```python
from build123d import *


with BuildPart() as part:
    # Sketch1 → Revolve1 (revolve)
    with BuildSketch(Plane.XY):
        with BuildLine():
            Line((18.654281973, 67.509460623), (18.654281973, 85.951651803))
            Line((18.654281973, 85.951651803), (14.554181768, 85.951651803))
            Line((14.554181768, 85.951651803), (14.554181768, 91.038742937))
            Line((14.554181768, 91.038742937), (18.654281973, 91.038742937))
            Line((18.654281973, 91.038742937), (18.654281973, 98.487697812))
            Line((18.654281973, 98.487697812), (14.554181768, 102.587798017))
            Line((14.554181768, 102.587798017), (18.654281973, 111.750471125))
            Line((18.654281973, 111.750471125), (-7.108349367, 111.750471125))
            Line((-7.108349367, 111.750471125), (-7.108349367, 98.487697812))
            Line((-7.108349367, 98.487697812), (7.996532166, 98.487697812))
            Line((7.996532166, 98.487697812), (7.996532166, 57.427605087))
            Line((7.996532166, 57.427605087), (0.444091399, 57.427605087))
            Line((0.444091399, 57.427605087), (0.444091399, 44.865685618))
            Line((0.444091399, 44.865685618), (4.926019535, 44.865685618))
            ThreePointArc((4.926019535, 44.865685618), (14.554181768, 54.511821478), (18.654281973, 67.509460623))
        make_face()
    revolve(axis=Axis((-7.108349367, 111.750471125, 0), (0, -1, 0)))

    # Sketch2 → Revolve2 (revolve)
    with BuildSketch(Plane(origin=(0, 85.951651803, 0), x_dir=(1, 0, 0), z_dir=(0, 1, 0))):
        Polygon((-12.941563399, -21.938938068), (-23.996434291, -19.455224522), (-36.865003284, -62.158981848), (-35.096912, -68.260719519), (-47.110720606, -71.741942645), (-42.631123157, -74.208704173), (-30.619424812, -70.728092534), (-32.80221788, -63.19520619), (-20.460781697, -37.558508231), (-17.141314342, -38.405147305), align=None)
    revolve(axis=Axis((-12.941563399, 85.951651803, 21.938938068), (-0.247140844, 0, 0.968979568)))


solid = part.part
```
CAD build for the part. Positions are in the model's coordinates, mm. A direction names the side the tool comes from. Round coordinates to 2 decimals unless told otherwise and drop trailing zeros. Use CSV: the item, a comma, the result in double quotes. Start each with the question number.
1) Saw through at A-A (y = 79.5). Count the separate pieces of the cut face and the enclosed holes in it, and give its area (3 significant figures).
2) Pin check, flat tips, straight feed: pin 1 Ø4 at (y, z) = (83.5, 18.5) entering from -X; pin 2 Ø10 at (y, z) = (91.5, 23.5) entering from -X; pin 3 Ø4 at (y, z) = (96.5, 15.5) entering from +X; pin 4 Ø9 at (x, z) = (-2.5, 4.5) entering from -Y. Stop position of each tip, or through.
3) Wall check: L1, parallel to Z at x = -16, y = 93.5; L2, parallel to Z at x = 1, y = 72.5; L3, parallel to Y at x = -18.5, z = -8.5. Give the ranges that are in metal, low to high. Write a range as [from, to].
4) Two-plate mould, pull along Z, no slides. Class faces 1 (the conical face through (-11.68, 85.24, 82.04)), 2 (the conical face through (-21.801, 82.356, 72.541)), 3 (the flat face through (-7, 111.75, 0)): pulls with the +Z half, pulls with the -Z half, needs draft (parallel to the pull), parting line crosses it, or undercut.
5) Tool access for faces 4 (the conical face through (-28.7, 81.23, 71.54)), 5 (the flat face through (0, 85.952, -21)): list every direction of +Z, -Z, +X, -X, +Y, -Y with a clear straight run to the whole face (end or side of a thin tool).
Values follow:
1,separate pieces,"1"
1,enclosed holes,"2"
1,area,"2,350 mm2"
2,pin 1,"stops at x = -26.89"
2,pin 2,"stops at x = -26.13"
2,pin 3,"stops at x = 14.83"
2,pin 4,"stops at y = 44.87"
3,L1,"z = [-24.18, -12.21], [12.21, 70.16], [74.69, 79.62]"
3,L2,"z = [-24.45, -12.74], [12.74, 24.45]"
3,L3,"y = [46.33, 57.43], [98.49, 111.75]"
4,face 1,"pulls with the +Z half"
4,face 2,"undercut"
4,face 3,"needs draft"
5,face 4,"+Z"
5,face 5,"none"
